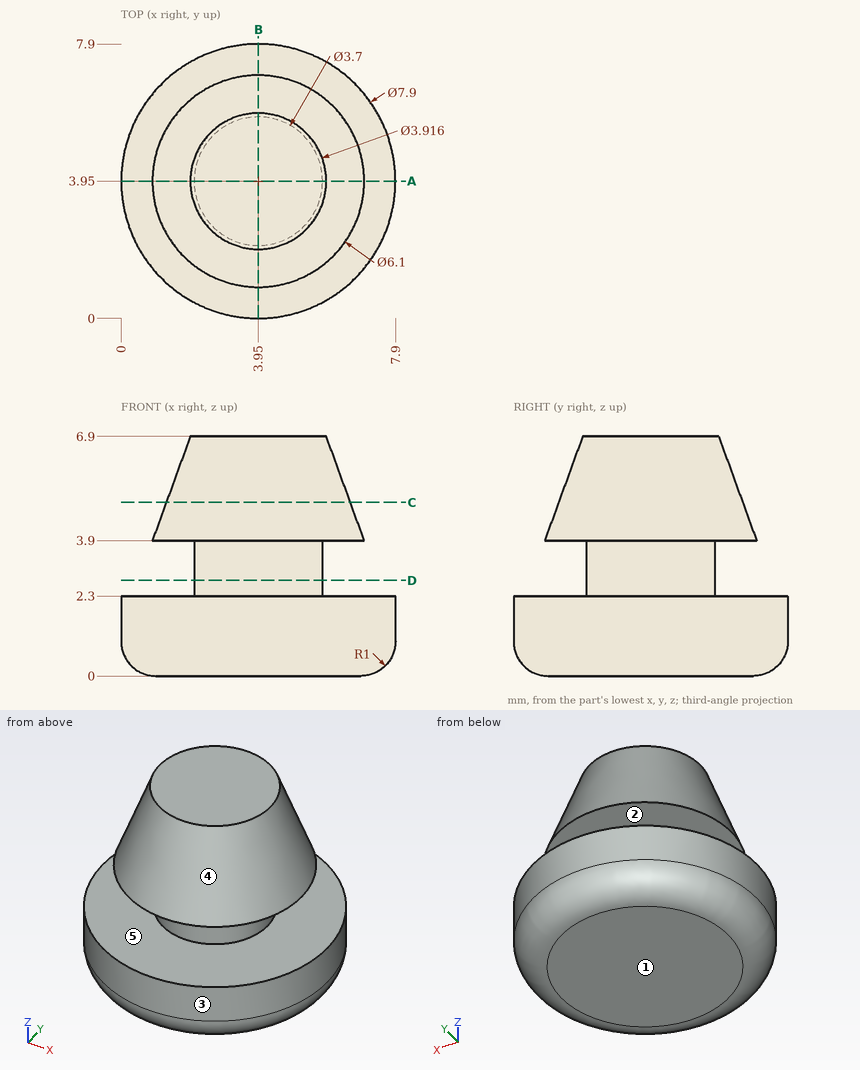
Could you check a few things on this drawing? It's one solid part, dimensions in mm from its lowest x, y, z. A direction names the side the tool comes from. Coordinates: 2 decimals unless noted, no trailing zeros. Order: outer loops, then holes, each group sorted by start corner. A loop starts at its lowest first (then second) coordinate and runs counter-clockwise, first axis right, second up.
1. If we section it at C-C (z = 5): Please give me the cut outline in (x, y).
2. Thinking about a two-plate mould opening in Z: for the marked faces 3, 4 and 5, which applies, +Z half, -Z half, draft (parallel to the pull), parting line (faces both ways), or undercut?
3. I need wall thicknesses on line 1 (Z direction, x = 5.25, y = 5.5); line 2 (Z direction, x = 2, y = 2.25); line 3 (Y direction, x = 5, z = 1.5). Which ranges of each line are inside material? Lowest first, please.
4. For the marked faces 1 and 2, which set-ups out of +Z, -Z, +X, -X, +Y, -Y let a thin tool reach every point of the face, with its end or its side?
5. If we section it at A-A (y = 3.95): Please give me the cut outline in (x, z).
6. If we section it at D-D (z = 2.75): Please give me the cut outline in (x, y).
7. I'm going to push flat-ended pins straight in: pin 1 (2 mm diameter, centred on x = 5, z = 1.5, fed in from -Y); pin 2 (3 mm diameter, centred on x = 1.5, z = 2, fed in from +Y); pin 3 (3 mm diameter, centred on y = 1.5, z = 5, fed in from -X); pin 4 (4 mm diameter, centred on y = 6.5, z = 3.5, fed in from +X). Where does each tip first touch, or does it pass through?
Entries:
1. outline: circle Ø5.3 at (3.95, 3.95)
2. face 3: draft
2. face 4: +Z half
2. face 5: undercut
3. line 1: z = 0 to 2.3, 3.9 to 6.72
3. line 2: z = 0 to 2.3, 3.9 to 5.17
3. line 3: y = 0.14 to 7.76
4. face 1: -Z, +X, -X, +Y, -Y
4. face 2: none
5. outline: (0, 1) arc R1 ccw to (1, 0) - (6.9, 0) arc R1 ccw to (7.9, 1) - (7.9, 2.3) - (5.8, 2.3) - (5.8, 3.9) - (7, 3.9) - (5.91, 6.9) - (1.99, 6.9) - (0.9, 3.9) - (2.1, 3.9) - (2.1, 2.3) - (0, 2.3) - close
6. outline: circle Ø3.7 at (3.95, 3.95)
7. pin 1: stops at y = 0
7. pin 2: stops at y = 7.78
7. pin 3: stops at x = 1.25
7. pin 4: stops at x = 7.78
